Work out the finished part from the listing and answer in its coordinate system (mm). A direction names the side the tool comes from. Round coordinates to 2 decimals unless told otherwise and drop trailing zeros. Write each loop counter-clockwise with the first axis right and the second up, starting at its lowest first coordinate (ties: lowest second). Pieces come first, ordered by that corner, then holes. Notation, with made-up numbers: M 11,-18 L 50,-18 A9 cw 50,-8 Z; hole C -22,33.5 d1. An arc over 180 degrees is marked long. One line per item, written item: value. Start each with the question number.
Q1. Find section D-D (y = -63). Write down the section's boundary in (x, z).
Q2. Find section C-C (z = 0). Write down the section's boundary in (x, y), and give its area (3 significant figures).
Q3. A tool of negligible diameter and unlimited length cuts with its end or side. For faces 5 (the cylindrical face through (32.923, -44.616, -33.774)), 6 (the flat face through (-38, -47, 18)), 7 (the flat face through (-28, -47, -28)), from which of +Z, -Z, +X, -X, +Y, -Y can it reach the whole face along a straight path? Write none if from no direction.
Q4. Consider probe 1 along Z at (x, y) = (-32, -70); probe 2 along Z at (x, y) = (-5, -64); probe 3 along Z at (x, y) = (0, -2.15). Determine where each line is inside the solid, lowest interval first.
Q5. Find section B-B (x = 0). Write down the section's boundary in (y, z), and give its area (3 significant figures).
Q6. The mould has two halves that part along X. Classify faces 1 (the flat face through (-28, -47, 28)), 2 (the flat face through (0, -43, -40)), 3 (the flat face through (38, -45, 37)), 4 (the cylindrical face through (-6, -6, 0)): released by +X, released by -X, zero draft, split by the parting line, or undercut.
Q7. Find section A-A (z = 32). Write down the section's boundary in (x, y), and give its area (3 significant figures).
Q8. Given pin 1 Ø2 at (x, z) = (-3.5, -25) entering from -Y; pin 2 Ø9 at (x, z) = (0, 0) entering from -Y; pin 3 Ø3 at (x, y) = (-38, -61) entering from +Z, each flat-ended and moving along its own axis, determine where each tip first touches the part or whether it passes through.
from build123d import *

# Parameters (mm, degrees)
F0_W      = 80
F0_H      = 80
F1_DEPTH  = 8
F2_R      = 4
F3_DEPTH  = 8.001
F5_DEPTH  = 80
F6_SIZE   = 5
F7_R      = 2
F8_DEPTH  = 88.001
F9_R      = 6
F10_DEPTH = 5


with BuildPart() as f1:
    # F0 (on Front) → F1 (new body)
    with BuildSketch(Plane.XZ):
        Rectangle(F0_W, F0_H)
    extrude(amount=F1_DEPTH)

    # F2 (on face) → F3 (cut, through all)
    with BuildSketch(Plane.XZ.offset(8)):
        Circle(F2_R)
    extrude(amount=-F3_DEPTH, mode=Mode.SUBTRACT)

    # F4 (on face) → F5 (join)
    with BuildSketch(Plane.XZ.offset(8)):
        Polygon((40, 40), (-40, 40), (-40, 18), (-36, 18), (-36, 20), (-20, 36), (20, 36), (36, 20), (36, 0), (36, -20), (20, -36), (-20, -36), (-36, -20), (-36, -18), (-40, -18), (-40, -40), (40, -40), align=None)
    extrude(amount=F5_DEPTH)

    # F6
    f6_edges = [f1.edges().sort_by_distance(p)[0] for p in [
        (-40, -44, 40),
        (40, -44, 40),
        (-40, -44, -40),
        (40, -44, -40),
    ]]
    chamfer(f6_edges, length=F6_SIZE)

    # F7 (on face) → F8 (cut, through all)
    with BuildSketch(Plane.XZ.offset(88)):
        with Locations((-32, 32)):
            Circle(F7_R)
        with Locations((-32, -32)):
            Circle(F7_R)
        with Locations((32, -32)):
            Circle(F7_R)
        with Locations((32, 32)):
            Circle(F7_R)
    extrude(amount=-F8_DEPTH, mode=Mode.SUBTRACT)

    # F9 (on face) → F10 (cut)
    with BuildSketch(Plane.XZ.offset(8)):
        Circle(F9_R)
    extrude(amount=-F10_DEPTH, mode=Mode.SUBTRACT)


solid = f1.part
The answers:
1. outline: M -40,-35 L -35,-40 L 35,-40 L 40,-35 L 40,35 L 35,40 L -35,40 L -40,35 L -40,18 L -36,18 L -36,20 L -20,36 L 20,36 L 36,20 L 36,-20 L 20,-36 L -20,-36 L -36,-20 L -36,-18 L -40,-18 Z; hole C -32,-32 d4; hole C -32,32 d4; hole C 32,-32 d4; hole C 32,32 d4
2. outline: M -40,-8 L -6,-8 L -6,-3 L -4,-3 L -4,0 L -40,0 Z; M 4,-3 L 6,-3 L 6,-8 L 36,-8 L 36,-88 L 40,-88 L 40,0 L 4,0 Z
2. area: 876 mm2
3. face 5: +Y, -Y
3. face 6: -X, -Y
3. face 7: -Y
4. probe 1: -40 to -34, -30 to -24, 24 to 30, 34 to 40
4. probe 2: -40 to -36, 36 to 40
4. probe 3: -40 to -4, 4 to 40
5. outline: M -88,-40 L 0,-40 L 0,-4 L -3,-4 L -3,-6 L -8,-6 L -8,-36 L -88,-36 Z; M -88,36 L -8,36 L -8,6 L -3,6 L -3,4 L 0,4 L 0,40 L -88,40 Z
5. area: 1,200 mm2
6. face 1: undercut
6. face 2: zero draft
6. face 3: released by +X
6. face 4: undercut
7. outline: M -40,-88 L -34,-88 L -34,0 L -40,0 Z; M -30,-88 L -24,-88 L -24,-8 L 24,-8 L 24,-88 L 30,-88 L 30,0 L -30,0 Z; M 34,-88 L 40,-88 L 40,0 L 34,0 Z
7. area: 2,500 mm2
8. pin 1: y = -8
8. pin 2: y = -3
8. pin 3: z = 38.5
